Model file for the job. Use its own axes, mm. Face numbers are marked on the shaded views. A direction names the side the tool comes from. Give positions to 0.01 mm unless a question says otherwise; leave off trailing zeros. Write each loop counter-clockwise with the first axis right and the second up, starting at its lowest first coordinate (ties: lowest second). Pieces come first, ordered by that corner, then holes. Notation, with made-up numbers: (-11.75, 14) - (19.25, 14) arc R24 cw to (19.25, 44) - close; hole circle Ø7 at (63, -17). An arc over 180 degrees is marked (long way). Use CSV: the item, a comma, the result in double quotes.
from build123d import *

# Parameters (mm, degrees)
F0_W     = 6
F0_H     = 3.175
F0_W_2   = 4
F1_DEPTH = 3.175


# Not quite as in the source:
# - a length typed as a fraction of an inch, garbled in the dataset ("3 / 203.2 mm" for 3/8 in), is restored


with BuildPart() as f1:
    # F0 (on Top) → F1 (new body)
    with BuildSketch(Plane.XY):
        Polygon((-26.613304615, 17.7200174183), (-26.613304615, 27.0450174183), (-30.613304615, 27.0450174183), (-36.613304615, 27.0450174183), (-36.613304615, -6.6049825817), (-26.613304615, -6.6049825817), (-22.613304615, -6.6049825817), (-19.613304615, -6.6049825817), (-19.613304615, 2.7200174183), (-21.113304615, 2.7200174183), (-21.113304615, 4.7200174183), (-19.613304615, 4.7200174183), (-19.613304615, 6.2200174183), (-16.613304615, 6.2200174183), (-16.613304615, 4.7200174183), (-15.113304615, 4.7200174183), (-15.113304615, 2.7200174183), (-16.613304615, 2.7200174183), (-16.613304615, -6.6049825817), (-13.613304615, -6.6049825817), (-9.613304615, -6.6049825817), (-9.613304615, 27.0450174183), (-13.613304615, 27.0450174183), (-19.613304615, 27.0450174183), (-23.613304615, 27.0450174183), (-23.613304615, 17.7200174183), (-22.113304615, 17.7200174183), (-22.113304615, 15.7200174183), (-23.613304615, 15.7200174183), (-23.613304615, 14.2200174183), (-26.613304615, 14.2200174183), (-26.613304615, 15.7200174183), (-28.113304615, 15.7200174183), (-28.113304615, 17.7200174183), align=None)
        with Locations((-33.613304615, 28.6325174183)):
            Rectangle(F0_W, F0_H)
        with Locations((-16.613304615, 28.6325174183)):
            Rectangle(F0_W, F0_H)
        with Locations((-24.613304615, -8.1924825817)):
            Rectangle(F0_W_2, F0_H)
        with Locations((-11.613304615, -8.1924825817)):
            Rectangle(F0_W_2, F0_H)
    extrude(amount=F1_DEPTH)


solid = f1.part
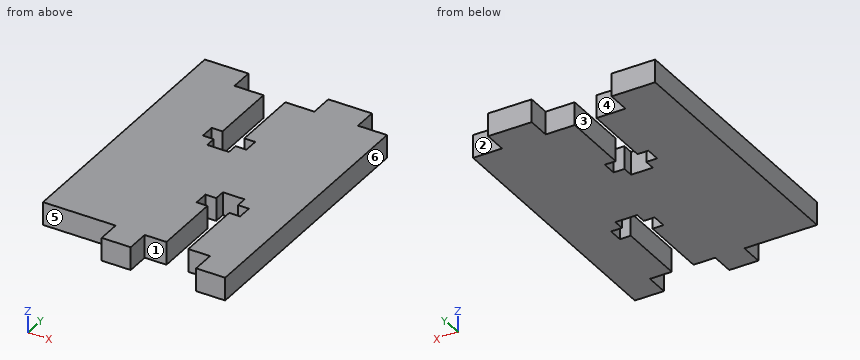
(1) Saw through at C-C, the plane x = -17.25. List the corners of the cut face in (y, z) (3 decimals), then the cut area to 3 significant figures.
Checked values:
outline,"(6.22, 0) - (30.22, 0) - (30.22, 3.175) - (6.22, 3.175) - close"
area,"76.2 mm^2"
(2) Saw through at A-A, the plane y = -6. List the corners of the cut face in (x, z) (3 decimals), then the cut area to 3 significant figures.
Checked values:
outline,"(-36.613, 0) - (-19.613, 0) - (-19.613, 3.175) - (-36.613, 3.175) - close; (-16.613, 0) - (-9.613, 0) - (-9.613, 3.175) - (-16.613, 3.175) - close"
area,"76.2 mm^2"
(3) Flat gauge pins, fed straight in: P1, Ø0.8, axis at x = -20.5, z = 1.5, coming from the -Y side (3 decimals); P2, Ø1.6, axis at x = -11, z = 2.5, coming from the +Y side (3 decimals); P3, Ø1, axis at y = -8, z = 1, coming from the -X side. Where does each tip first touch, or does it go through?
Checked values:
P1,"stops at y = -6.605"
P2,"stops at y = 27.045"
P3,"stops at x = -26.61"
(4) Pull direction X, two halves, no side cores. Call the marked faces 4, 5 and 6: released by +X, released by -X, zero draft, split by the parting line, or undercut.
Checked values:
face 4,"undercut"
face 5,"zero draft"
face 6,"released by +X"
(5) 3-axis set-ups, long thin cutter, end or side, ignore diameter. For the marked faces 1, 2 and 3: which of +Z, -Z, +X, -X, +Y, -Y reach the whole face in a straight line?
Checked values:
face 1,"+Z, -Z, -Y"
face 2,"+Z, -Z, +X, +Y"
face 3,"+Z, -Z, +Y"
(6) Wall check: probe 1 along X at (y, z) = (24, 2.1); probe 2 along Y at (x, z) = (-22.5, 1.95); probe 3 along Y at (x, z) = (-22.75, 2.25). Give the ranges that are in metal, low to high. Write a range as [from, to].
Checked values:
probe 1,"x = [-36.61, -26.61], [-23.61, -9.61]"
probe 2,"y = [-6.6, 15.72], [17.72, 27.05]"
probe 3,"y = [-9.78, 15.72], [17.72, 27.05]"
(7) Saw through at B-B, the plane x = -32.25. List the corners of the cut face in (y, z) (3 decimals), then the cut area to 3 significant figures.
Checked values:
outline,"(-6.605, 0) - (30.22, 0) - (30.22, 3.175) - (-6.605, 3.175) - close"
area,"117 mm^2"
